Geometry: final body of the model. Coordinates: model frame, mm. Give positions to 0.01 mm unless a question says otherwise; leave off trailing zeros.
1. First-contact query: P1, Ø11, axis at x = 215.51, z = 44.23, coming from the +Y side; P2, Ø1.5, axis at x = -39.5, y = -3.5, coming from the +Z side. Flat tips, straight axial feed; report the tip coordinate or a pass-through.
2. Section A-A, the plane y = -2.25. State how many separate pieces and enclosed holes the cut face has, then the cut area to 3 significant figures.
3. Material intervals for line 1 along X through (y, z) = (-1, 43); line 2 along X through (y, z) = (-4.8, 95); line 3 along Z through (x, y) = (-196, -1.5), sorted ascending.
from build123d import *

# Parameters (mm, degrees)
F0_R     = 240
F0_R_2   = 6
F1_DEPTH = 5
F2_SIZE  = 1
F3_SIZE  = 1


with BuildPart() as f1:
    # F0 (on Front) → F1 (new body)
    with BuildSketch(Plane.XZ):
        with Locations((9.9e-05, -1.9e-05)):
            Circle(F0_R)
        with Locations((-148.349302, -162.457568)):
            Circle(F0_R_2, mode=Mode.SUBTRACT)
        with Locations((-24.526936, -218.628527)):
            Circle(F0_R_2, mode=Mode.SUBTRACT)
        with Locations((-215.507239, -44.233347)):
            Circle(F0_R_2, mode=Mode.SUBTRACT)
        with Locations((108.663924, -191.290827)):
            Circle(F0_R_2, mode=Mode.SUBTRACT)
        with Locations((200.348896, -90.88654)):
            Circle(F0_R_2, mode=Mode.SUBTRACT)
        with Locations((-200.030377, 90.541344)):
            Circle(F0_R_2, mode=Mode.SUBTRACT)
        with Locations((-108.663725, 191.290789)):
            Circle(F0_R_2, mode=Mode.SUBTRACT)
        with Locations((215.507437, 44.233309)):
            Circle(F0_R_2, mode=Mode.SUBTRACT)
        with Locations((23.815236, 219.336878)):
            Circle(F0_R_2, mode=Mode.SUBTRACT)
        with Locations((148.3495, 162.45753)):
            Circle(F0_R_2, mode=Mode.SUBTRACT)
    extrude(amount=F1_DEPTH)

    # F2
    f2_edges = [f1.edges().sort_by_distance(p)[0] for p in [
        (-239.999901, -5, -1.9e-05),
        (-154.349302, -5, -162.457568),
        (-30.526936, -5, -218.628527),
        (-221.507239, -5, -44.233347),
        (102.663924, -5, -191.290827),
        (194.348896, -5, -90.88654),
        (-206.030377, -5, 90.541344),
        (-114.663725, -5, 191.290789),
        (209.507437, -5, 44.233309),
        (17.815236, -5, 219.336878),
        (142.3495, -5, 162.45753),
    ]]
    chamfer(f2_edges, length=F2_SIZE)

    # F3
    f3_edges = [f1.edges().sort_by_distance(p)[0] for p in [
        (-239.999901, 0, -1.9e-05),
        (-154.349302, 0, -162.457568),
        (-30.526936, 0, -218.628527),
        (-221.507239, 0, -44.233347),
        (102.663924, 0, -191.290827),
        (194.348896, 0, -90.88654),
        (-206.030377, 0, 90.541344),
        (-114.663725, 0, 191.290789),
        (209.507437, 0, 44.233309),
        (17.815236, 0, 219.336878),
        (142.3495, 0, 162.45753),
    ]]
    chamfer(f3_edges, length=F3_SIZE)


solid = f1.part
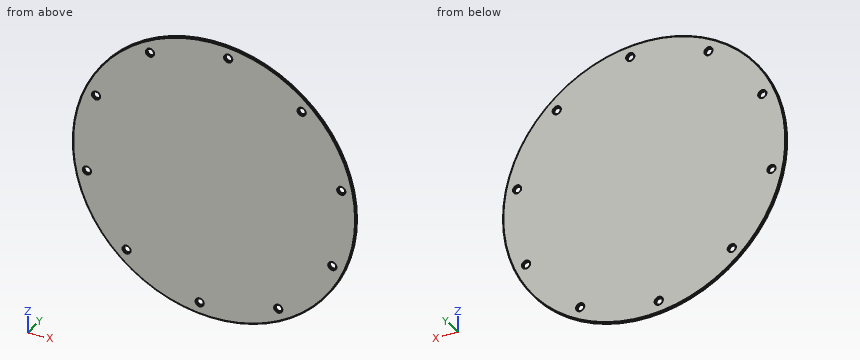
Answers below:
1. P1: passes through
1. P2: stops at z = 236.85
2. separate pieces: 1
2. enclosed holes: 10
2. area: 180,000 mm2
3. line 1: x = -236.12 to 209.64, 221.38 to 236.12
3. line 2: x = -219.53 to -205.16, -194.9 to 219.53
3. line 3: z = -138.51 to 86.1, 94.99 to 138.51
